Geometry check sheet. Reference: the model listing, model coordinates, mm. A direction names the side the tool comes from. Coordinates: 2 decimals unless noted, no trailing zeros. Order: outer loops, then holes, each group sorted by start corner. A loop starts at its lowest first (then second) coordinate and runs counter-clockwise, first axis right, second up. Notation, with made-up numbers: (62, 53.25) - (103, 53.25) arc R25 ccw to (103, 75.25) - close; hole circle Ø10 at (41, 87.25). An arc over 180 degrees is marked (long way). One line per item, written item: value. Start each with the question number.
```python
from build123d import *

# Parameters (mm, degrees)
F1_DEPTH = 25.4


with BuildPart() as f1:
    # F0 (on Front) → F1 (new body)
    with BuildSketch(Plane.XZ):
        Polygon((68.58, -20.32), (76.2, -12.7), (60.96, -12.7), align=None)
        Polygon((60.96, -12.7), (76.2, -12.7), (76.2, 12.7), (-76.2, 12.7), (-76.2, -12.7), (-60.96, -12.7), (-45.72, -12.7), (-30.48, -12.7), (-15.24, -12.7), (0, -12.7), (15.24, -12.7), (30.48, -12.7), (45.72, -12.7), align=None)
        Polygon((53.34, -20.32), (60.96, -12.7), (45.72, -12.7), align=None)
        Polygon((38.1, -20.32), (45.72, -12.7), (30.48, -12.7), align=None)
        Polygon((22.86, -20.32), (30.48, -12.7), (15.24, -12.7), align=None)
        Polygon((-60.96, -12.7), (-76.2, -12.7), (-68.58, -20.32), align=None)
        Polygon((7.62, -20.32), (15.24, -12.7), (0, -12.7), align=None)
        Polygon((-45.72, -12.7), (-60.96, -12.7), (-53.34, -20.32), align=None)
        Polygon((-7.62, -20.32), (0, -12.7), (-15.24, -12.7), align=None)
        Polygon((-30.48, -12.7), (-45.72, -12.7), (-38.1, -20.32), align=None)
        Polygon((-22.86, -20.32), (-15.24, -12.7), (-30.48, -12.7), align=None)
    extrude(amount=F1_DEPTH)


solid = f1.part
```
Q1. Material ranges on probe 1 along Z at (x, y) = (30.5, -4.25); probe 2 along Z at (x, y) = (54.5, -22.75), recorded low to high.
Q2. Set-up check for faces 5 (the flat face through (3.8, -12.5, -16.5)), 6 (the flat face through (76.2, -13, 0)): record each of +Z, -Z, +X, -X, +Y, -Y from which the full face is reachable in a straight line by a thin tool's end or side.
Q3. Gauge pin test, flat ends, axial feed: P1, Ø8, axis at x = 9, y = -21, coming from the -Z side; P2, Ø6, axis at x = 60, y = -18.5, coming from the -Z side; P3, Ø2, axis at x = -35, z = -12.5, coming from the +Y side; P4, Ø10, axis at x = -13.5, y = -7.5, coming from the -Z side. Record the tip position at first contact, or that the pin passes through.
Q4. Cross-section at B-B, the plane z = -15.5. Count the separate pieces of the cut face and the enclosed holes in it, and give its area (3 significant figures).
Q5. Cross-section at C-C, the plane x = -51. Enter the section's corners in (y, z).
Q6. Cross-section at D-D, the plane x = 26.5. Enter the section's corners in (y, z).
Q7. Release check for a two-part mould opening along X. For faces 1 (the flat face through (-11.48, -12.52, -16.46)), 2 (the flat face through (1, -13, 12.7)), 3 (the flat face through (-76.2, -13, 0)), 4 (the flat face through (-26.72, -12.52, -16.46)) record: released by +X, released by -X, zero draft, split by the parting line, or undercut.
Q8. Cross-section at A-A, the plane y = -16.75. Enter the section's corners in (x, z), and give its area (3 significant figures).
Check result:
1. probe 1: z = -12.72 to 12.7
1. probe 2: z = -19.16 to 12.7
2. face 5: -Z, +Y, -Y
2. face 6: +Z, -Z, +X, +Y, -Y
3. P1: stops at z = -20.32
3. P2: stops at z = -16.66
3. P3: stops at y = 0
3. P4: stops at z = -19.44
4. separate pieces: 10
4. enclosed holes: 0
4. area: 2,450 mm2
5. outline: (-25.4, -17.98) - (0, -17.98) - (0, 12.7) - (-25.4, 12.7) - close
6. outline: (-25.4, -16.68) - (0, -16.68) - (0, 12.7) - (-25.4, 12.7) - close
7. face 1: undercut
7. face 2: zero draft
7. face 3: released by -X
7. face 4: undercut
8. outline: (-76.2, -12.7) - (-68.58, -20.32) - (-60.96, -12.7) - (-53.34, -20.32) - (-45.72, -12.7) - (-38.1, -20.32) - (-30.48, -12.7) - (-22.86, -20.32) - (-15.24, -12.7) - (-7.62, -20.32) - (0, -12.7) - (7.62, -20.32) - (15.24, -12.7) - (22.86, -20.32) - (30.48, -12.7) - (38.1, -20.32) - (45.72, -12.7) - (53.34, -20.32) - (60.96, -12.7) - (68.58, -20.32) - (76.2, -12.7) - (76.2, 12.7) - (-76.2, 12.7) - close
8. area: 4,450 mm2
